Check sheet for the drawn part. Datum: minimum x, y, z corner. Units: mm. Round coordinates to 2 decimals unless told otherwise and drop trailing zeros. Write each loop counter-clockwise with the first axis right and the second up, starting at its lowest first coordinate (ties: lowest second). Pieces come first, ordered by that corner, then holes. Notation, with made-up numbers: (-25, -27.5) - (33, -27.5) arc R19 cw to (33, 9.5) - close; hole circle Ø5 at (60, -29.75). An arc over 180 degrees is marked (long way). Answer as a JSON object with one key per item and string values. Group by question number.
Item 1: Thickness scan on line 1 (X direction, y = 13, z = 42) (1 decimal); line 2 (X direction, y = 34, z = 46) (1 decimal); line 3 (Z direction, x = 118, y = 4). Record the ranges inside material, lowest first.
Item 2: Sectioned sample at A-A on x = 19. Record the boundary of the cut face in (y, z).
Item 3: Gauge pin test, flat end, axial feed: P1, Ø23, axis at x = 114.11, z = 41.88, coming from the +Y side. Record the tip position at first contact, or that the pin passes through.
Item 4: Release check for a two-part mould opening along Z. For the marked faces 1, 2 and 3 record: pulls with the +Z half, pulls with the -Z half, needs draft (parallel to the pull), parting line crosses it, or undercut.
Item 5: Sectioned sample at B-B on z = 24.5. Record the boundary of the cut face in (x, y) (1 decimal), plus the area to 3 significant figures.
Item 6: Sectioned sample at D-D on x = 38. Record the boundary of the cut face in (y, z).
Item 7: Sectioned sample at C-C on y = 26.5. Count the separate pieces of the cut face and the enclosed holes in it, plus the area to 3 significant figures.
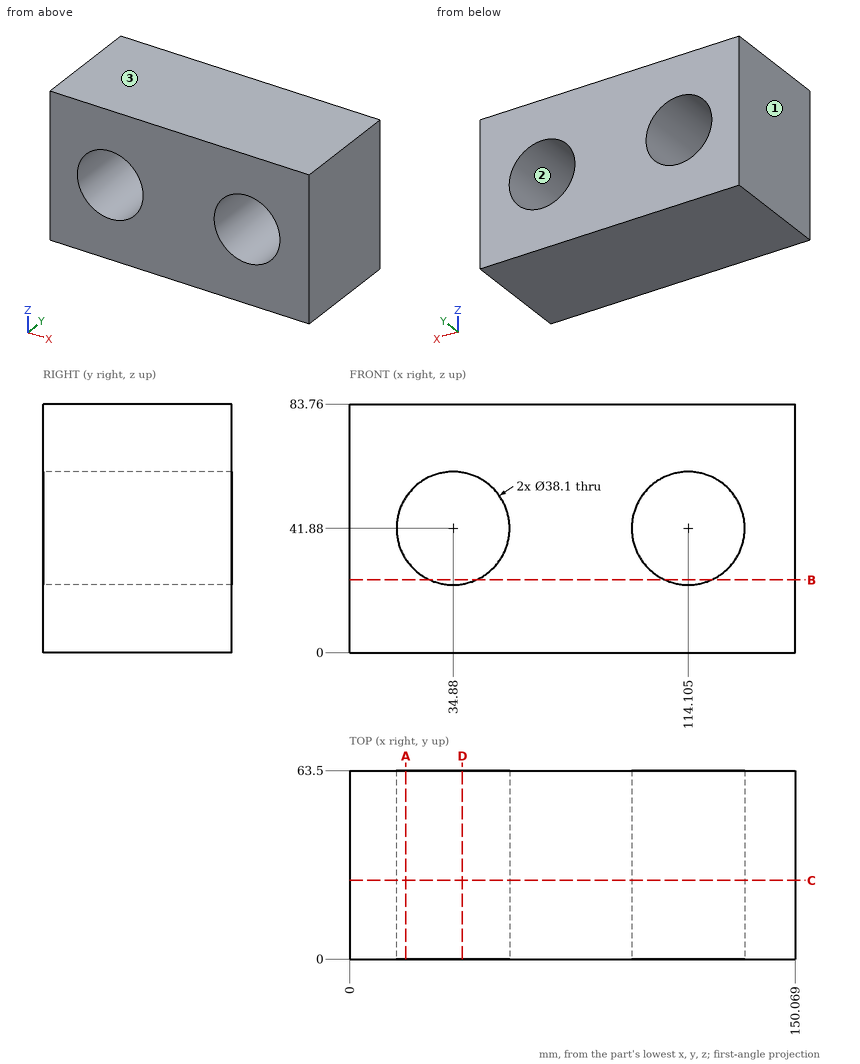
Completed:
{
 "1": {"line 1": "0 to 15.8, 53.9 to 95.1, 133.2 to 150.1", "line 2": "0 to 16.3, 53.5 to 95.5, 132.7 to 150.1", "line 3": "0 to 23.23, 60.53 to 83.76"},
 "2": {"outline": "(0, 0) - (63.5, 0) - (63.5, 31.36) - (0, 31.36) - close; (0, 52.4) - (63.5, 52.4) - (63.5, 83.76) - (0, 83.76) - close"},
 "3": {"P1": "through"},
 "4": {"face 1": "needs draft", "face 2": "undercut", "face 3": "pulls with the +Z half"},
 "5": {"outline": "(0, 0) - (27.1, 0) - (27.1, 63.5) - (0, 63.5) - close; (42.7, 0) - (106.3, 0) - (106.3, 63.5) - (42.7, 63.5) - close; (121.9, 0) - (150.1, 0) - (150.1, 63.5) - (121.9, 63.5) - close", "area": "7,550 mm²"},
 "6": {"outline": "(0, 0) - (63.5, 0) - (63.5, 23.09) - (0, 23.09) - close; (0, 60.67) - (63.5, 60.67) - (63.5, 83.76) - (0, 83.76) - close"},
 "7": {"separate pieces": "1", "enclosed holes": "2", "area": "10,300 mm²"}
}
